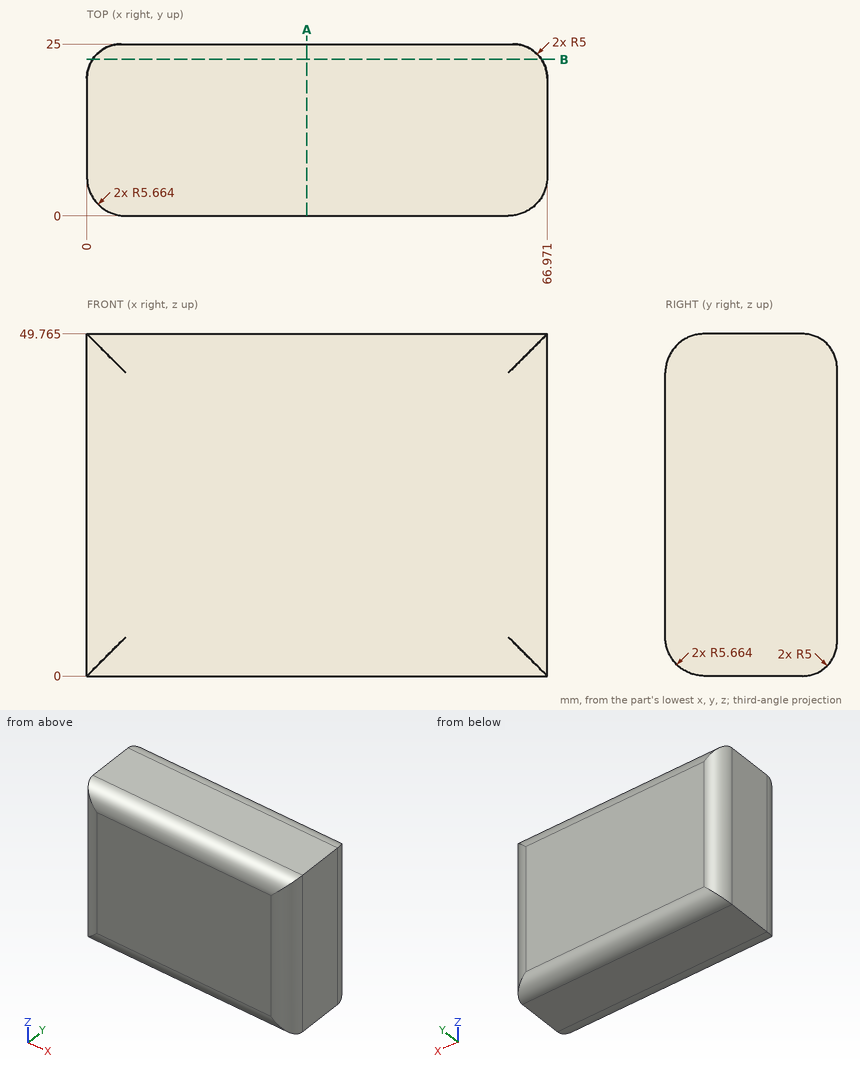
Design review of the part shown in the three views and the two pictorial views. Dimensions are in mm from the part's minimum x, y and z. Give positions to 0.01 mm unless a question says otherwise; leave off trailing zeros. Loops run counter-clockwise (first coordinate to the right, second up) from the corner with the lowest first, then second, coordinate; pieces in that order, holes last. Notation, with made-up numbers: M 12.5,-5.5 L 68.5,-5.5 A18 cw 68.5,17.5 Z; hole C 77,-31 d9. An arc over 180 degrees is marked long. Answer as a JSON object with one key per item and string values. Group by question number.
Q1. Add section A-A on x = 32. Give the boundary of the cut face in (y, z) (1 decimal).
Q2. For probe 1 along X at (y, z) = (20.25, 44) (1 decimal); probe 2 along Y at (x, z) = (7, 46.5); probe 3 along Z at (x, y) = (62, 23) (1 decimal), list the stretches that pass through material, from the lowest coordinate up. Write a range as [from, to].
Q3. Insertion check: P1, Ø1, axis at x = 16.5, y = 20.5, coming from the -Z side; P2, Ø5, axis at x = 28, y = 3, coming from the +Z side. Each pin has a flat end and moves straight along its axis. Give the tip position at first contact, or say it passes through.
Q4. Add section B-B on y = 22.75. Give the boundary of the cut face in (x, z) (1 decimal), and give its area (3 significant figures).
Checked values:
{
 "1": {"outline": "M 0,5.7 A5.7 ccw 5.7,0 L 20,0 A5 ccw 25,5 L 25,44.8 A5 ccw 20,49.8 L 5.7,49.8 A5.7 ccw 0,44.1 Z"},
 "2": {"probe 1": "[0, 67]", "probe 2": "[0.53, 24.69]", "probe 3": "[1, 48.8]"},
 "3": {"P1": "z = 0", "P2": "z = 49.76"},
 "4": {"outline": "M 0.8,0.8 L 66.1,0.8 L 66.1,48.9 L 0.8,48.9 Z", "area": "3,140 mm²"}
}
